Verification items for the finished model (mm, model axes). Face numbers are marked on the shaded views. A direction names the side the tool comes from. Coordinates: 2 decimals unless noted, no trailing zeros. Order: outer loops, then holes, each group sorted by start corner. A loop starts at its lowest first (then second) coordinate and runs counter-clockwise, first axis right, second up. Notation, with made-up numbers: M 34,84 L 83,84 A15 ccw 83,94 Z; hole C 46.5,16 d5. An arc over 180 degrees is marked long. Write item = value, one per line.
```python
from build123d import *

# Parameters (mm, degrees)
SKETCH1_W           = 106.68
SKETCH1_H           = 147.32
BOSS_EXTRUDE1_DEPTH = 38.1
SHELL1_T            = -5.08
SKETCH5_R           = 0.889
SKETCH5_W           = 3.302
SKETCH5_H           = 25.908
SKETCH5_W_2         = 25.4
SKETCH5_H_2         = 5.842
CUT_EXTRUDE1_DEPTH  = 38.1
CUT_EXTRUDE2_DEPTH  = 107.68
SKETCH15_R          = 2.54
BOSS_EXTRUDE5_DEPTH = 5.08


with BuildPart() as part:
    # Sketch1 → Boss-Extrude1 (new body)
    with BuildSketch(Plane(origin=(0, 0, 0), x_dir=(1, 0, 0), z_dir=(0, 1, 0))):
        Rectangle(SKETCH1_W, SKETCH1_H)
    extrude(amount=BOSS_EXTRUDE1_DEPTH)

    # Shell1
    shell1_openings = [part.faces().sort_by_distance(p)[0] for p in [
        (0, 0, 0),
    ]]
    offset(amount=SHELL1_T, openings=shell1_openings, kind=Kind.INTERSECTION)

    # Sketch5 → Cut-Extrude1 (cut)
    with BuildSketch(Plane(origin=(0, 38.1, 0), x_dir=(1, 0, 0), z_dir=(0, 1, 0))):
        with Locations((-25.4, 51.435)):
            Circle(SKETCH5_R)
        with Locations((-25.4, 22.225)):
            Circle(SKETCH5_R)
        with Locations((25.4, 36.83)):
            Rectangle(SKETCH5_W, SKETCH5_H)
        with Locations((25.4, 51.435)):
            Circle(SKETCH5_R)
        with Locations((25.4, 22.225)):
            Circle(SKETCH5_R)
        with Locations((0, -63.119)):
            Rectangle(SKETCH5_W_2, SKETCH5_H_2)
        with Locations((29.845, -60.198)):
            Circle(SKETCH5_R)
        with Locations((-29.845, -60.198)):
            Circle(SKETCH5_R)
        with Locations((-29.845, -1.016)):
            Circle(SKETCH5_R)
        with Locations((29.845, -1.016)):
            Circle(SKETCH5_R)
    extrude(amount=-CUT_EXTRUDE1_DEPTH, mode=Mode.SUBTRACT)

    # Sketch6 → Cut-Extrude2 (cut, through all)
    with BuildSketch(Plane.ZY.offset(53.34)):
        with BuildLine():
            Line((-63.5, -17.421133293), (-63.5, 5.08))
            ThreePointArc((-63.5, 5.08), (-58.42, 10.16), (-53.34, 5.08))
            Line((-53.34, 5.08), (-53.34, -17.421133293))
            ThreePointArc((-53.34, -17.421133293), (-58.42, -22.501133293), (-63.5, -17.421133293))
        make_face()
    extrude(amount=-CUT_EXTRUDE2_DEPTH, mode=Mode.SUBTRACT)

    # Sketch15 → Boss-Extrude5 (add)
    with BuildSketch(Plane.XZ):
        with BuildLine():
            Line((-53.34, -73.66), (-53.34, -78.74))
            ThreePointArc((-53.34, -78.74), (-48.26, -83.82), (-43.18, -78.74))
            Line((-43.18, -78.74), (-43.18, -73.66))
            Line((-43.18, -73.66), (-53.34, -73.66))
        make_face()
        with Locations((-48.26, -78.74)):
            Circle(SKETCH15_R, mode=Mode.SUBTRACT)
        with BuildLine():
            Line((53.34, -73.66), (43.18, -73.66))
            Line((43.18, -73.66), (43.18, -78.74))
            ThreePointArc((43.18, -78.74), (48.26, -83.82), (53.34, -78.74))
            Line((53.34, -78.74), (53.34, -73.66))
        make_face()
        with Locations((48.26, -78.74)):
            Circle(SKETCH15_R, mode=Mode.SUBTRACT)
        with BuildLine():
            Line((43.18, 78.74), (43.18, 73.66))
            Line((43.18, 73.66), (53.34, 73.66))
            Line((53.34, 73.66), (53.34, 78.74))
            ThreePointArc((53.34, 78.74), (48.26, 83.82), (43.18, 78.74))
        make_face()
        with Locations((48.26, 78.74)):
            Circle(SKETCH15_R, mode=Mode.SUBTRACT)
        with BuildLine():
            Line((-53.34, 78.74), (-53.34, 73.66))
            Line((-53.34, 73.66), (-43.18, 73.66))
            Line((-43.18, 73.66), (-43.18, 78.74))
            ThreePointArc((-43.18, 78.74), (-48.26, 83.82), (-53.34, 78.74))
        make_face()
        with Locations((-48.26, 78.74)):
            Circle(SKETCH15_R, mode=Mode.SUBTRACT)
    extrude(amount=-BOSS_EXTRUDE5_DEPTH)


solid = part.part
```
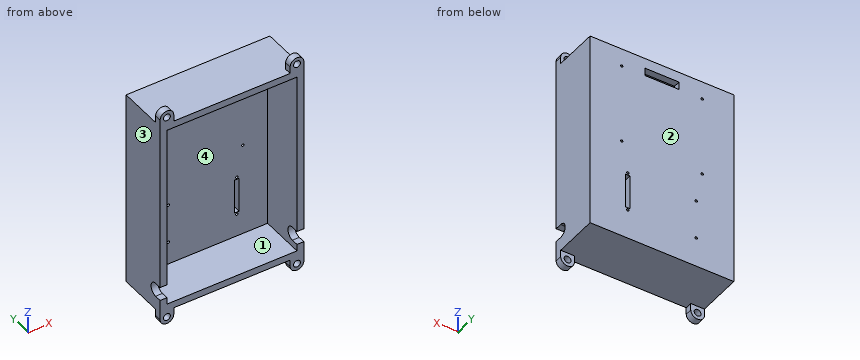
Item 1: Sectioned sample at C-C, the plane z = -58.42. Enter the section's corners in (x, y).
Report:
outline = M -53.34,10.16 L -48.26,10.16 L -48.26,33.02 L 48.26,33.02 L 48.26,10.16 L 53.34,10.16 L 53.34,38.1 L -53.34,38.1 Z
Item 2: Gauge pin test, flat ends, axial feed: pin 1 (6 mm diameter, centred on x = 48.26, z = 78.74, fed in from +Y); pin 2 (1.5 mm diameter, centred on x = 1, z = 29, fed in from -Y); pin 3 (11.5 mm diameter, centred on x = -19.5, y = 13.5, fed in from -Z). Record the tip position at first contact, or that the pin passes through.
Report:
pin_1 = 5.08
pin_2 = 33.02
pin_3 = -73.66
Item 3: Tool access check on the marked faces 3 and 4. Record the directions out of +Z, -Z, +X, -X, +Y, -Y that give a thin tool (end or side, any length) a straight path to the whole face; none if there is none.
Report:
face_3 = +Z, -Z, -X, +Y, -Y
face_4 = -Y
Item 4: Sectioned sample at A-A, the plane y = 8.5. Enter the section's corners in (x, z).
Report:
outline = M -53.34,-73.66 L 53.34,-73.66 L 53.34,-62.18 L 48.26,-62.18 L 48.26,-68.58 L -48.26,-68.58 L -48.26,-62.18 L -53.34,-62.18 Z; M -53.34,-54.66 L -48.26,-54.66 L -48.26,68.58 L 48.26,68.58 L 48.26,-54.66 L 53.34,-54.66 L 53.34,73.66 L -53.34,73.66 Z
Item 5: Release check for a two-part mould opening along Z. For the marked faces 1 and 2 record: pulls with the +Z half, pulls with the -Z half, needs draft (parallel to the pull), parting line crosses it, or undercut.
Report:
face_1 = undercut
face_2 = needs draft
Item 6: Sectioned sample at D-D, the plane x = 20.5. Enter the section's corners in (y, z), then the cut area to 3 significant figures.
Report:
outline = M 0,-73.66 L 38.1,-73.66 L 38.1,73.66 L 0,73.66 L 0,68.58 L 33.02,68.58 L 33.02,-68.58 L 0,-68.58 Z
area = 1,080 mm^2
Item 7: Sectioned sample at B-B, the plane x = -10.5. Enter the section's corners in (y, z), then the cut area to 3 significant figures.
Report:
outline = M 0,-73.66 L 38.1,-73.66 L 38.1,60.2 L 33.02,60.2 L 33.02,-68.58 L 0,-68.58 Z; M 0,68.58 L 33.02,68.58 L 33.02,66.04 L 38.1,66.04 L 38.1,73.66 L 0,73.66 Z
area = 1,050 mm^2
Item 8: Scan lines: L1, parallel to X at y = 12.5, z = -15.5; L2, parallel to X at y = 34, z = -32; L3, parallel to Z at x = 40.5, y = 10. Record each from-to range of solid material in increasing order. Write a range as from..to.
Report:
L1 = -53.34..-48.26, 48.26..53.34
L2 = -53.34..23.75, 27.05..53.34
L3 = -73.66..-68.58, 68.58..73.66
